Read the model definition and answer for the solid it produces. Units are mm, in the model's axes. A direction names the side the tool comes from. Coordinates: 2 decimals unless noted, no trailing zeros. Write each loop counter-clockwise with the first axis right and the second up, starting at its lowest first coordinate (ties: lowest second). Pieces come first, ordered by that corner, then holes. Notation, with made-up numbers: M -32,6.5 L -5,6.5 A17 ccw -5,36.5 Z; hole C -9,-15.5 d9. An arc over 180 degrees is marked long. Write item = value, one per line.
from build123d import *

# Parameters (mm, degrees)
F0_W     = 37
F0_H     = 17
F1_DEPTH = 0.8
F2_W     = 21.1
F2_H     = 8.5
F3_DEPTH = 6.9
F4_R     = 1.5
F5_R     = 0.5


with BuildPart() as f1:
    # F0 (on Top) → F1 (new body)
    with BuildSketch(Plane.XY):
        Rectangle(F0_W, F0_H)
    extrude(amount=F1_DEPTH)

    # F2 (on face) → F3 (join)
    with BuildSketch(Plane.XY.offset(0.8)):
        with Locations((7.95, 4.25)):
            Rectangle(F2_W, F2_H)
        with Locations((7.95, -4.25)):
            Rectangle(F2_W, F2_H)
    extrude(amount=F3_DEPTH)

    # F4
    f4_edges = [f1.edges().sort_by_distance(p)[0] for p in [
        (18.5, -8.5, 3.85),
        (18.5, 8.5, 3.85),
        (-2.6, 8.5, 4.25),
        (-2.6, -8.5, 4.25),
    ]]
    fillet(f4_edges, radius=F4_R)

    # F5
    f5_edges = [f1.edges().sort_by_distance(p)[0] for p in [
        (7.95, 8.5, 7.7),
    ]]
    fillet(f5_edges, radius=F5_R)


solid = f1.part
Item 1: Which of the six approach directions +Z, -Z, +X, -X, +Y, -Y give full straight-line access (tool end or side, diameter ignored) to faces 1 (the face through (-2.6, 0, 4)), 2 (the face through (-2.17, -8.05, 4.04)), 3 (the face through (-2.17, 8.05, 4.04))?
Worked answers:
face_1 = +Z, -X, +Y, -Y
face_2 = +Z, -X, -Y
face_3 = +Z, -X, +Y
Item 2: Find section B-B (z = 2.25). Determine the outline of the cut face in (x, y).
Worked answers:
outline = M -2.6,-7 A1.5 ccw -1.1,-8.5 L 17,-8.5 A1.5 ccw 18.5,-7 L 18.5,7 A1.5 ccw 17,8.5 L -1.1,8.5 A1.5 ccw -2.6,7 Z
Item 3: Find section C-C (x = -5). Determine the outline of the cut face in (y, z), and give its area (3 significant figures).
Worked answers:
outline = M -8.5,0 L 8.5,0 L 8.5,0.8 L -8.5,0.8 Z
area = 13.6 mm²
Item 4: Flat-ended cylindrical pins translate along their axes: pin 1 (1 mm diameter, centred on y = -1.5, z = 5.5, fed in from -X); pin 2 (5 mm diameter, centred on x = -11, y = 3.5, fed in from +Z). Find the tip coordinate at first contact, or state that the pin passes through.
Worked answers:
pin_1 = -2.6
pin_2 = 0.8
Item 5: Consider line 1 along X through (y, z) = (2.5, 5.5); line 2 along Z through (x, y) = (-3.5, 3); line 3 along Y through (x, z) = (16, 7.25). Determine where each line is inside the solid, lowest interval first. Write a range as from..to.
Worked answers:
line_1 = -2.6..18.5
line_2 = 0..0.8
line_3 = -8.5..8.5
Item 6: Find section A-A (y = 6.5). Determine the outline of the cut face in (x, z), and give its area (3 significant figures).
Worked answers:
outline = M -18.5,0 L 18.5,0 L 18.5,7.2 A0.5 ccw 18,7.7 L -2.1,7.7 A0.5 ccw -2.6,7.2 L -2.6,0.8 L -18.5,0.8 Z
area = 175 mm²
